Can you work these out from the drawing? Everything is in mm from the part's minimum corner. A direction names the side the tool comes from. Give positions to 0.01 mm unless a question says otherwise; leave off trailing zeros. Order: outer loops, then holes, each group sorted by start corner. A loop starts at its lowest first (then second) coordinate and runs counter-clockwise, first axis right, second up. Notation, with made-up numbers: (-1.5, 51) -> (21.5, 51) arc R26 cw to (21.5, 72) -> close; hole circle Ø9 at (-12.5, 58). An arc over 180 degrees is marked (long way). Answer as CSV lines item,"result". Start each with the question number.
(1) I want a section at C-C (z = 6.25). Please give me the cut outline in (x, y).
(2) I want a section at D-D (x = 8). Please give me the cut outline in (y, z), plus the area to 3 significant figures.
(3) I want a section at A-A (x = 4.5). Please give me the cut outline in (y, z).
(4) I need wall thicknesses on L1, parallel to Y at x = 4.5, z = 8.5; L2, parallel to Z at x = 1.5, y = 6.25; L3, parallel to X at y = 6.25, z = 8.5. Which ranges of each line are inside material? Lowest first, please.
(5) Will these pins go through, and if not, where does the flat tip stop? pin 1 Ø2.5 at (x, y) = (2.5, 6) entering from -Z; pin 2 Ø1.5 at (x, z) = (3, 1.5) entering from +Y.
(6) We'd pull the mould along X, two halves only. Please class the marked faces 3, 4 and 5: released by +X, released by -X, zero draft, split by the parting line, or undercut.
(7) On a 3-axis mill with a long thin cutter (end or side, diameter ignored), from which of +Z, -Z, +X, -X, +Y, -Y can I reach the whole of each face in a straight line? I mean the marked faces 1 and 2. Say none if no direction works.
(8) I want a section at B-B (y = 4.5). Please give me the cut outline in (x, z).
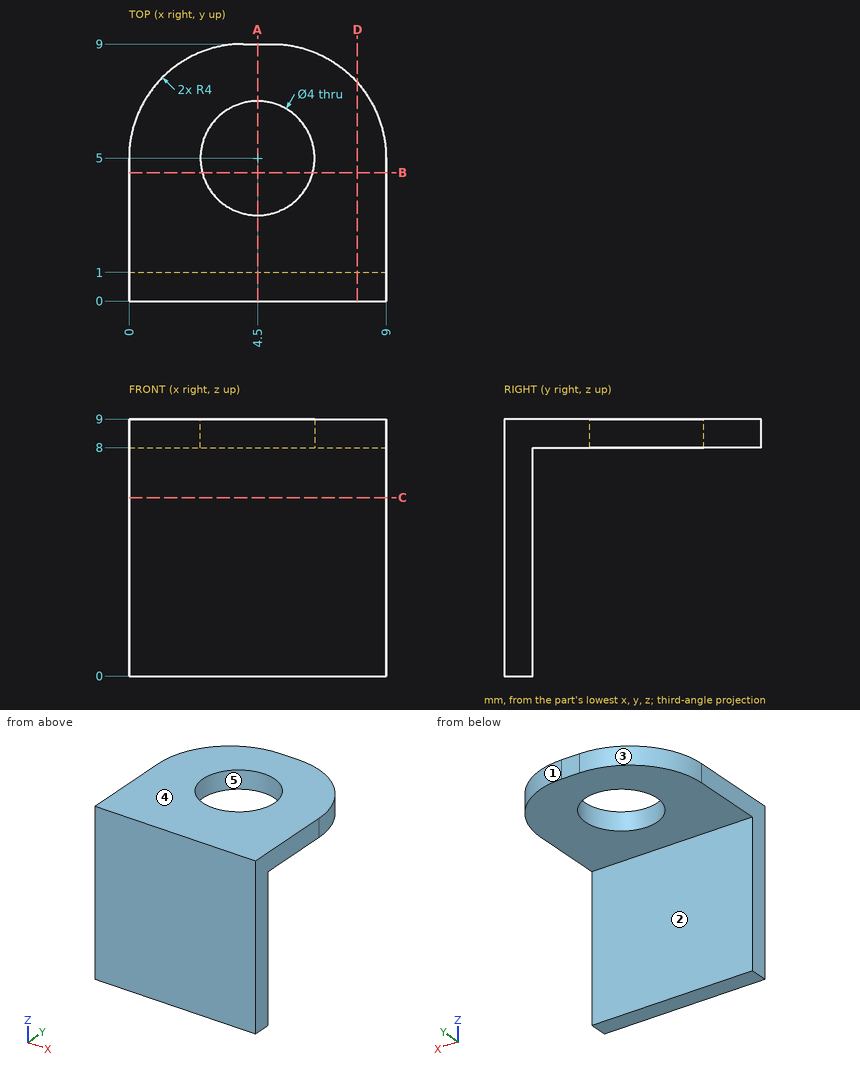
Final values:
1,outline,"(0, 0) -> (9, 0) -> (9, 1) -> (0, 1) -> close"
2,outline,"(0, 0) -> (1, 0) -> (1, 8) -> (7.65, 8) -> (7.65, 9) -> (0, 9) -> close"
2,area,"15.6 mm²"
3,outline,"(0, 0) -> (1, 0) -> (1, 8) -> (3, 8) -> (3, 9) -> (0, 9) -> close; (7, 8) -> (9, 8) -> (9, 9) -> (7, 9) -> close"
4,L1,"0 to 3, 7 to 9"
4,L2,"8 to 9"
4,L3,"0.2 to 2.94, 6.06 to 8.8"
5,pin 1,"z = 8"
5,pin 2,"y = 1"
6,face 3,"released by -X"
6,face 4,"zero draft"
6,face 5,"undercut"
7,face 1,"+Z, -Z, +X, +Y"
7,face 2,"-Z, +X, -X, +Y"
8,outline,"(0, 8) -> (2.56, 8) -> (2.56, 9) -> (0, 9) -> close; (6.44, 8) -> (9, 8) -> (9, 9) -> (6.44, 9) -> close"
